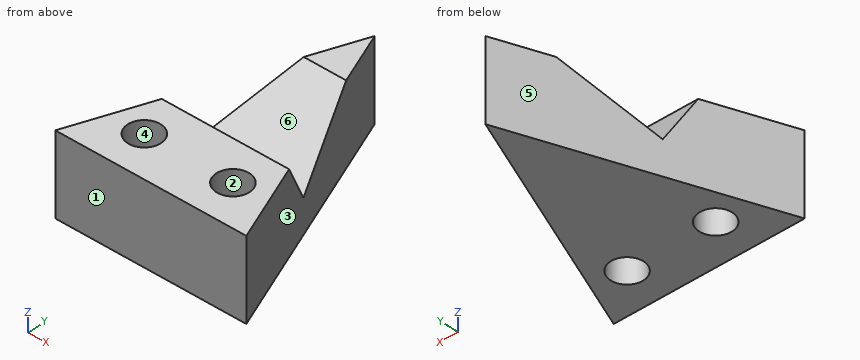
```python
from build123d import *

# Parameters (mm, degrees)
F0_R     = 7.874
F1_DEPTH = 38.1
F4_DEPTH = 89.408


with BuildPart() as f1:
    # F0 (on Top) → F1 (new body)
    with BuildSketch(Plane.XY):
        Polygon((0, 57.15), (-44.704, -57.15), (44.704, -57.15), align=None)
        with Locations((-20.738764, -37.846)):
            Circle(F0_R, mode=Mode.SUBTRACT)
        with Locations((20.738764, -37.846)):
            Circle(F0_R, mode=Mode.SUBTRACT)
    extrude(amount=F1_DEPTH)

    # F3 (on offset) → F4 (cut)
    with BuildSketch(Plane.YZ.offset(44.704)):
        Polygon((31.75, 38.1), (-19.05, 38.1), (-6.35, 16.102955), align=None)
    extrude(amount=-F4_DEPTH, mode=Mode.SUBTRACT)


solid = f1.part
```
Could you check a few things on this model? Use its own coordinates, in mm. Face numbers are marked on the shaded views. A direction names the side the tool comes from. Give positions to 0.01 mm unless a question says otherwise; leave off trailing zeros. Loops run counter-clockwise (first coordinate to the right, second up) from the corner with the lowest first, then second, coordinate; pieces in that order, holes last. Notation, with made-up numbers: (14.25, 55.5) -> (70.25, 55.5) arc R26 cw to (70.25, 89.5) -> close; hole circle Ø6 at (27.25, 75). An arc over 180 degrees is marked (long way). Put each result on its own line as item: value.
(1) Imagine slicing it at A-A on z = 27.5. Write out the boundary of the cut face in (x, y), plus the area to 3 significant figures.
Computed:
outline: (-44.7, -57.15) -> (44.7, -57.15) -> (27.41, -12.93) -> (-27.41, -12.93) -> close; (-17.11, 13.39) -> (17.11, 13.39) -> (0, 57.15) -> close; hole circle Ø15.75 at (-20.74, -37.85); hole circle Ø15.75 at (20.74, -37.85)
area: 3,550 mm^2
(2) I'm going to push flat-ended pins straight in: pin 1 Ø10 at (x, y) = (17.5, -10.5) entering from -Z; pin 2 Ø1.5 at (y, z) = (-23, 21.5) entering from +X; pin 3 Ø8 at (y, z) = (23.5, 25) entering from +X; pin 4 Ø10 at (y, z) = (-38, 12.5) entering from +X. Where does each tip first touch, or does it pass through?
Computed:
pin 1: z = 0
pin 2: x = 31.64
pin 3: x = 14.73
pin 4: x = 39.17
(3) Imagine slicing it at B-B on x = -16.5. Write out the boundary of the cut face in (y, z), plus the area to 3 significant figures.
Computed:
outline: (-57.15, 0) -> (-44.48, 0) -> (-44.48, 38.1) -> (-57.15, 38.1) -> close; (-31.21, 0) -> (14.96, 0) -> (14.96, 28.41) -> (-6.35, 16.1) -> (-19.05, 38.1) -> (-31.21, 38.1) -> close
area: 1,760 mm^2
(4) Thinking about a two-plate mould opening in X: for the marked faces 1, 2, 3 and 4, which applies, pulls with the +X half, pulls with the -X half, needs draft (parallel to the pull), parting line crosses it, or undercut?
Computed:
face 1: needs draft
face 2: undercut
face 3: pulls with the +X half
face 4: undercut
(5) For the marked faces 5 and 6, which set-ups out of +Z, -Z, +X, -X, +Y, -Y let a thin tool reach every point of the face, with its end or its side?
Computed:
face 5: +Z, -Z, -X, +Y
face 6: +Z, +X, -X
(6) Please list where these lines run through material, in increasing order: probe 1 along Y at (x, z) = (-20, 27.5); probe 2 along Y at (x, z) = (18, 32); probe 3 along X at (y, z) = (29, 24). Write a range as [from, to].
Computed:
probe 1: [-57.15, -45.69], [-30.01, -12.93]
probe 2: [-57.15, -45.23], [-30.46, -15.53]
probe 3: [-11.01, 11.01]
(7) Imagine slicing it at C-C on z = 14. Write out the boundary of the cut face in (x, y), plus the area to 3 significant figures.
Computed:
outline: (-44.7, -57.15) -> (44.7, -57.15) -> (0, 57.15) -> close; hole circle Ø15.75 at (-20.74, -37.85); hole circle Ø15.75 at (20.74, -37.85)
area: 4,720 mm^2
(8) Imagine slicing it at D-D on x = 21. Write out the boundary of the cut face in (y, z).
Computed:
outline: (-57.15, 0) -> (-45.72, 0) -> (-45.72, 38.1) -> (-57.15, 38.1) -> close; (-29.98, 0) -> (3.46, 0) -> (3.46, 21.76) -> (-6.35, 16.1) -> (-19.05, 38.1) -> (-29.98, 38.1) -> close
